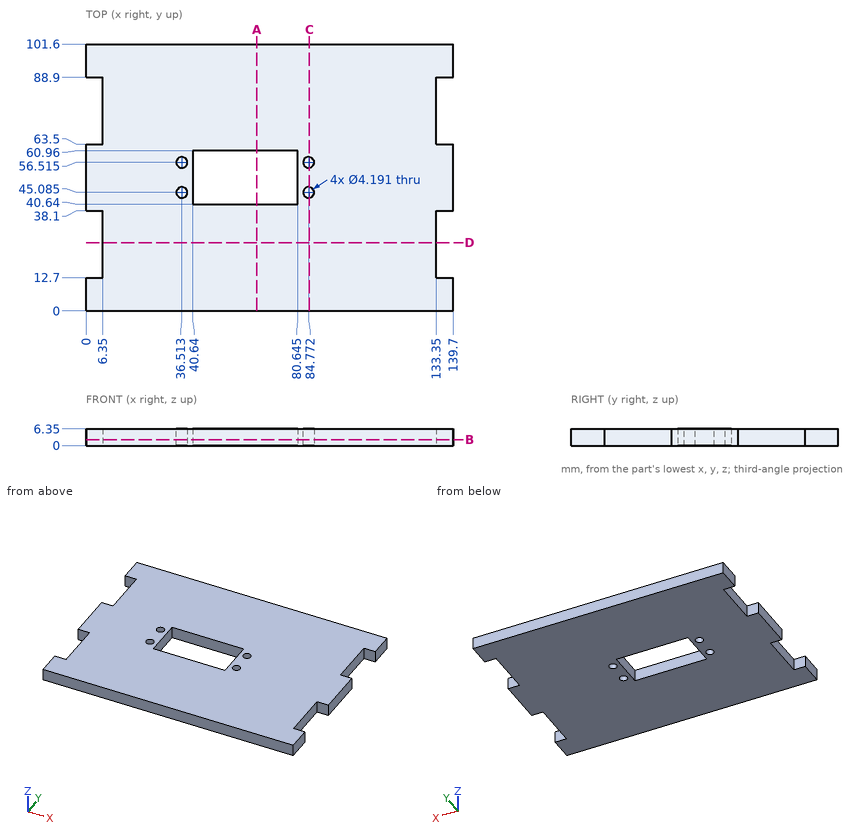
The figure shows three views and two pictorial views of one solid part (mm, origin at its lowest corner). Answer the questions. Round coordinates to 2 decimals unless told otherwise and drop trailing zeros. Order: outer loops, then holes, each group sorted by start corner. A loop starts at its lowest first (then second) coordinate and runs counter-clockwise, first axis right, second up. Notation, with made-up numbers: (56.5, -6.5) -> (94.5, -6.5) arc R24 cw to (94.5, 12.5) -> close; hole circle Ø2 at (43, 35.5). An arc over 180 degrees is marked (long way). Put each result on its own line as item: value.
Q1. Each of these flat-tipped pins is pushed along its axis until it touches: P1, Ø1.5, axis at y = 19, z = 2, coming from the +X side; P2, Ø2, axis at x = 94, z = 3, coming from the -Y side. Where does it stop, or does it pass through?
Results list:
P1: x = 133.35
P2: y = 0
Q2. Section C-C, the plane x = 85 is taken. Write down the section's boundary in (y, z), and give its area (3 significant figures).
Results list:
outline: (0, 0) -> (43, 0) -> (43, 6.35) -> (0, 6.35) -> close; (47.17, 0) -> (54.43, 0) -> (54.43, 6.35) -> (47.17, 6.35) -> close; (58.6, 0) -> (101.6, 0) -> (101.6, 6.35) -> (58.6, 6.35) -> close
area: 592 mm^2
Q3. Consider line 1 along Y through (x, z) = (42.5, 5.5); line 2 along X through (y, z) = (50.5, 2.5) (1 decimal); line 3 along X through (y, z) = (18, 2.5). Determine where each line is inside the solid, lowest interval first.
Results list:
line 1: 0 to 40.64, 60.96 to 101.6
line 2: 0 to 40.6, 80.6 to 139.7
line 3: 6.35 to 133.35
Q4. Section D-D, the plane y = 26 is taken. Write down the section's boundary in (x, z).
Results list:
outline: (6.35, 0) -> (133.35, 0) -> (133.35, 6.35) -> (6.35, 6.35) -> close
Q5. Section B-B, the plane z = 2.25 is taken. Count the separate pieces of the cut face and the enclosed holes in it, and give its area (3 significant figures).
Results list:
separate pieces: 1
enclosed holes: 5
area: 12,700 mm^2
Q6. Section A-A, the plane x = 65 is taken. Write down the section's boundary in (y, z).
Results list:
outline: (0, 0) -> (40.64, 0) -> (40.64, 6.35) -> (0, 6.35) -> close; (60.96, 0) -> (101.6, 0) -> (101.6, 6.35) -> (60.96, 6.35) -> close
